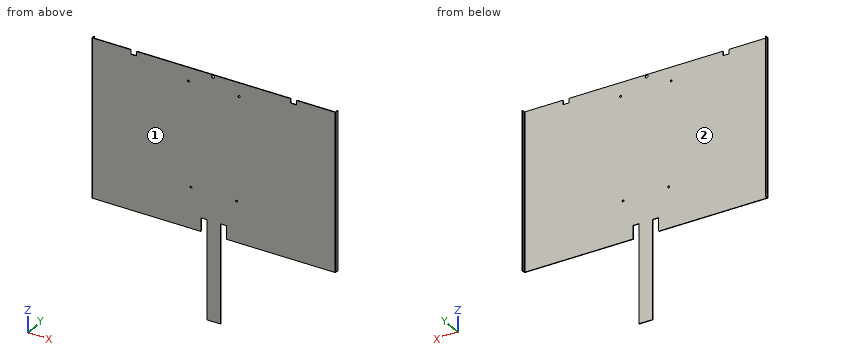
```python
from build123d import *

# Parameters (mm, degrees)
SM_BASE_FLANGE_1_DEPTH             = 2
SM_EDGE_FLANGE_1_STRIP_W           = 9.48
SM_EDGE_FLANGE_1_STRIP_H           = 2
SM_EDGE_FLANGE_1_STRIP_CUT_DEPTH   = 530.740059044
SM_EDGE_FLANGE_1_STRIP_2_W         = 9.48
SM_EDGE_FLANGE_1_STRIP_2_H         = 2
SM_EDGE_FLANGE_1_STRIP_CUT_2_DEPTH = 530.740059044
SM_EDGE_FLANGE_1_DEPTH             = 530.740059044
SM_EDGE_FLANGE_1_BEND_DEPTH        = 530.740059044
SKETCH_12_R                        = 5
CUT_EXTRUDE_1_DEPTH                = 3
SKETCH_13_R                        = 3.25
CUT_EXTRUDE_2_DEPTH                = 5


# Read off the part's stored shape, not the designer's step: Базовая кромка1
# Sheet-metal steps are written as plain solids
with BuildPart() as part:
    # Базовая кромка1 outline → Базовая кромка1 (new body)
    with BuildSketch(Plane(origin=(0, 0, 0), x_dir=(1, 0, 0), z_dir=(0, 1, 0))):
        Polygon((-23, -331.526743508), (-43, -331.526743508), (-43, -286.526743508), (-410, -286.526743508), (-410, -817.266802552), (-279.163690552, -817.266802552), (-279.163690552, -802.266802552), (-259.163690552, -802.266802552), (-259.163690552, -817.266802552), (259.163690552, -817.266802552), (259.163690552, -802.266802552), (279.163690552, -802.266802552), (279.163690552, -817.266802552), (410, -817.266802552), (410, -286.526743508), (43, -286.526743508), (43, -331.526743508), (23, -331.526743508), (23, 0), (-23, 0), align=None)
    extrude(amount=SM_BASE_FLANGE_1_DEPTH)

    # Ребро-кромка1 strip (across the edge) → Ребро-кромка1 strip cut (cut)
    with BuildSketch(Plane(origin=(410, 2, 817.266802552), x_dir=(-1, 0, 0), z_dir=(0, 0, -1))):
        with Locations((-2, -1)):
            Rectangle(SM_EDGE_FLANGE_1_STRIP_W, SM_EDGE_FLANGE_1_STRIP_H)
    extrude(amount=SM_EDGE_FLANGE_1_STRIP_CUT_DEPTH, mode=Mode.SUBTRACT)

    # Ребро-кромка1 strip 2 (across the edge) → Ребро-кромка1 strip cut 2 (cut)
    with BuildSketch(Plane(origin=(-410, 2, 286.526743508), x_dir=(1, 0, 0), z_dir=(0, 0, 1))):
        with Locations((-2, -1)):
            Rectangle(SM_EDGE_FLANGE_1_STRIP_2_W, SM_EDGE_FLANGE_1_STRIP_2_H)
    extrude(amount=SM_EDGE_FLANGE_1_STRIP_CUT_2_DEPTH, mode=Mode.SUBTRACT)

    # Ребро-кромка1 section (across the edge) → Ребро-кромка1 (add)
    with BuildSketch(Plane(origin=(410, 2, 817.266802552), x_dir=(-1, 0, 0), z_dir=(0, 0, -1))):
        with BuildLine():
            Line((0, 0.74), (0, 10))
            Line((0, 10), (2, 10))
            Line((2, 10), (2, 0.74))
            ThreePointArc((2, 0.74), (2.216740982, 0.216740982), (2.74, 0))
            Line((2.74, 0), (2.74, -2))
            ThreePointArc((2.74, -2), (0.80252742, -1.19747258), (0, 0.74))
        make_face()
    extrude(amount=SM_EDGE_FLANGE_1_DEPTH)

    # Ребро-кромка1 section 2 (across the edge) → Ребро-кромка1 bend (add)
    with BuildSketch(Plane(origin=(-410, 2, 286.526743508), x_dir=(1, 0, 0), z_dir=(0, 0, 1))):
        with BuildLine():
            Line((0, 0.74), (0, 10))
            Line((0, 10), (2, 10))
            Line((2, 10), (2, 0.74))
            ThreePointArc((2, 0.74), (2.216740982, 0.216740982), (2.74, 0))
            Line((2.74, 0), (2.74, -2))
            ThreePointArc((2.74, -2), (0.80252742, -1.19747258), (0, 0.74))
        make_face()
    extrude(amount=SM_EDGE_FLANGE_1_BEND_DEPTH)

    # Эскиз12 → Вырез-Вытянуть1 (cut)
    with BuildSketch(Plane(origin=(0, 2, 0), x_dir=(1, 0, 0), z_dir=(0, 1, 0))):
        with Locations(Location((-2.5, -811.266802552, 0), (0, 0, 270))):
            Circle(SKETCH_12_R)
    extrude(amount=-CUT_EXTRUDE_1_DEPTH, mode=Mode.SUBTRACT)

    # Эскиз13 → Вырез-Вытянуть2 (cut)
    with BuildSketch(Plane(origin=(0, 2, 0), x_dir=(1, 0, 0), z_dir=(0, 1, 0))):
        with Locations(Location((76.777184185, -422.982246008, 0), (0, 0, 270))):
            Circle(SKETCH_13_R)
        with Locations(Location((85.329382087, -771.621076737, 0), (0, 0, 270))):
            Circle(SKETCH_13_R)
        with Locations(Location((-85.329382087, -771.621076737, 0), (0, 0, 270))):
            Circle(SKETCH_13_R)
        with Locations(Location((-76.777184185, -422.982246008, 0), (0, 0, 270))):
            Circle(SKETCH_13_R)
    extrude(amount=-CUT_EXTRUDE_2_DEPTH, mode=Mode.SUBTRACT)


solid = part.part
```
Verification items for the finished model (mm, model axes). Face numbers are marked on the shaded views. Round coordinates to 2 decimals unless told otherwise and drop trailing zeros. Order: outer loops, then holes, each group sorted by start corner. A loop starts at its lowest first (then second) coordinate and runs counter-clockwise, first axis right, second up.
1) Material ranges on line 1 (X direction, y = 3, z = 649.5); line 2 (Y direction, x = 126, z = 729); line 3 (Z direction, x = -216.5, y = 0.5), recorded low to high.
Geometry says:
line 1: x = -410 to -408, 408 to 410
line 2: y = 0 to 2
line 3: z = 286.53 to 817.27
2) Draft check along X on the marked faces 1 and 2. Enter one of: +X half, -X half, draft (parallel to the pull), parting line (faces both ways), or undercut.
Geometry says:
face 1: draft
face 2: undercut
3) Cross-section at B-B, the plane z = 664. Record the cut outline in (x, y).
Geometry says:
outline: (-410, 2.74) arc R2.74 ccw to (-407.26, 0) - (407.26, 0) arc R2.74 ccw to (410, 2.74) - (410, 12) - (408, 12) - (408, 2.74) arc R0.74 cw to (407.26, 2) - (-407.26, 2) arc R0.74 cw to (-408, 2.74) - (-408, 12) - (-410, 12) - close
4) Cross-section at A-A, the plane y = 9. Record the cut outline in (x, z).
Geometry says:
outline: (-410, 286.53) - (-408, 286.53) - (-408, 817.27) - (-410, 817.27) - close; (408, 286.53) - (410, 286.53) - (410, 817.27) - (408, 817.27) - close
5) Depth check by flat-ended pin: pin 1 (13 mm diameter, centred on x = -2.5, z = 811.27, fed in from +Y); pin 2 (1 mm diameter, centred on x = -274, y = 1.5, fed in from +Z); pin 3 (4 mm diameter, centred on y = 3.5, z = 224, fed in from -X); pin 4 (4 mm diameter, centred on x = 76.78, z = 422.98, fed in from -Y). Enter the tip coordinate at first touch or a pass-through.
Geometry says:
pin 1: stops at y = 2
pin 2: stops at z = 802.27
pin 3: stops at x = -23
pin 4: passes through
6) Cross-section at C-C, the plane x = 172.5. Record the cut outline in (y, z), plus the area to 3 significant figures.
Geometry says:
outline: (0, 286.53) - (2, 286.53) - (2, 817.27) - (0, 817.27) - close
area: 1,060 mm2
